```python
from build123d import *

# Parameters (mm, degrees)
SKETCH2_W           = 112
SKETCH2_H           = 60
SKETCH2_W_2         = 20
SKETCH2_H_2         = 3
SKETCH2_W_3         = 3
SKETCH2_H_3         = 15
BOSS_EXTRUDE1_DEPTH = 3
SKETCH4_W           = 20
SKETCH4_H           = 3
CUT_EXTRUDE2_DEPTH  = 10


with BuildPart() as part:
    # Sketch2 → Boss-Extrude1 (new body)
    with BuildSketch(Plane.XY):
        Rectangle(SKETCH2_W, SKETCH2_H)
        with Locations((-35, -31.5)):
            Rectangle(SKETCH2_W_2, SKETCH2_H_2)
        with Locations((0, -31.5)):
            Rectangle(SKETCH2_W_2, SKETCH2_H_2)
        with Locations((35, -31.5)):
            Rectangle(SKETCH2_W_2, SKETCH2_H_2)
        with Locations((57.5, -15)):
            Rectangle(SKETCH2_W_3, SKETCH2_H_3)
        with Locations((-57.5, -15)):
            Rectangle(SKETCH2_W_3, SKETCH2_H_3)
        with Locations((-57.5, 15)):
            Rectangle(SKETCH2_W_3, SKETCH2_H_3)
        with Locations((57.5, 15)):
            Rectangle(SKETCH2_W_3, SKETCH2_H_3)
    extrude(amount=BOSS_EXTRUDE1_DEPTH)

    # Sketch4 → Cut-Extrude2 (cut)
    with BuildSketch(Plane.XY.offset(3)):
        with Locations((-35, 6)):
            Rectangle(SKETCH4_W, SKETCH4_H)
        with Locations((0, 6)):
            Rectangle(SKETCH4_W, SKETCH4_H)
        with Locations((35, 6)):
            Rectangle(SKETCH4_W, SKETCH4_H)
        Polygon((-59, 22.5), (-59, 7.5), (-56, 7.5), (-45, 7.5), (-25, 7.5), (-10, 7.5), (10, 7.5), (25, 7.5), (45, 7.5), (56, 7.5), (59, 7.5), (59, 22.5), (56, 22.5), (56, 30), (-56, 30), (-56, 22.5), align=None)
    extrude(amount=-CUT_EXTRUDE2_DEPTH, mode=Mode.SUBTRACT)


solid = part.part
```
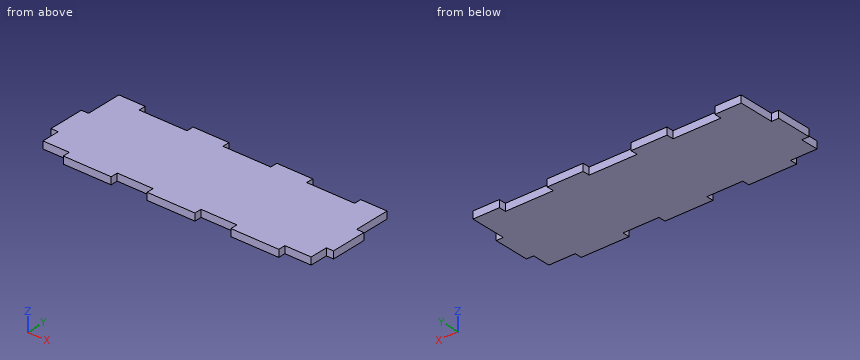
Could you check a few things on this model? Use its own coordinates, in mm. Give positions to 0.01 mm unless a question says otherwise; leave off trailing zeros. Loops run counter-clockwise (first coordinate to the right, second up) from the corner with the lowest first, then second, coordinate; pieces in that order, holes last. Notation, with made-up numbers: (82.25, 26.25) - (114.25, 26.25) arc R14 cw to (114.25, 40.25) - close; hole circle Ø4 at (31.25, 20). An arc over 180 degrees is marked (long way). Answer in a Markdown table with one row per item. Add a question column.
Q1. Please list where these lines run through material, in increasing order: L1, parallel to Y at x = 49.5, z = 1.25; L2, parallel to Y at x = 27.5, z = 1.45; L3, parallel to X at y = -6, z = 1.05. Write a range as from..to.
Q2. If we section it at A-A (y = 5.5): List the corners of the cut face in (x, z) for me, plus the area to 3 significant figures.
Q3. If we section it at B-B (x = -36): List the corners of the cut face in (y, z) for me.
Q4. For pin 1 (1.5 mm diameter, centred on x = 4.5, z = 2, fed in from +Y); pin 2 (1.5 mm diameter, centred on y = -31.5, z = 1.5, fed in from -X); pin 3 (1.5 mm diameter, centred on y = -24.5, z = 2, fed in from +X), each with a flat end and sliding along its axis, tell me the tip position at first contact or that it passes through.
Q5. If we section it at C-C (y = -1): List the corners of the cut face in (x, z) for me.
The answers:
| question | item | result |
|---|---|---|
| 1 | L1 | y = -30..7.5 |
| 1 | L2 | y = -33..4.5 |
| 1 | L3 | x = -56..56 |
| 2 | outline | (-56, 0) - (-45, 0) - (-45, 3) - (-56, 3) - close; (-25, 0) - (-10, 0) - (-10, 3) - (-25, 3) - close; (10, 0) - (25, 0) - (25, 3) - (10, 3) - close; (45, 0) - (56, 0) - (56, 3) - (45, 3) - close |
| 2 | area | 156 mm^2 |
| 3 | outline | (-33, 0) - (4.5, 0) - (4.5, 3) - (-33, 3) - close |
| 4 | pin 1 | stops at y = 4.5 |
| 4 | pin 2 | stops at x = -45 |
| 4 | pin 3 | stops at x = 56 |
| 5 | outline | (-56, 0) - (56, 0) - (56, 3) - (-56, 3) - close |
